The model under review builds one solid part; all positions refer to its coordinate system, in mm. A direction names the side the tool comes from. Coordinates: 2 decimals unless noted, no trailing zeros. Order: outer loops, then holes, each group sorted by start corner. A loop starts at its lowest first (then second) coordinate and runs counter-clockwise, first axis right, second up. Notation, with made-up numbers: (33, 20) -> (63, 20) arc R19 cw to (63, 33) -> close; hole circle Ø2 at (35, 63.5). An arc over 180 degrees is marked (long way). Use one line per item in the form item = value. Start each with the question number.
(1) Take a section at A-A (y = 15.5). State the section outline as (x, z) points, then the cut area to 3 significant figures.
(2) Take a section at D-D (y = 10.25). State the section outline as (x, z) points.
(3) Wall thickness on line 1 along Y through (x, z) = (-21, 2.3); line 2 along X through (y, z) = (0, 1.9); line 3 along X through (y, z) = (-3.5, 1.65): over which ranges is each line inside the solid? List them lowest first.
(4) Take a section at C-C (x = -6). State the section outline as (y, z) points.
(5) Take a section at B-B (z = 1.85). State the section outline as (x, y) points.
(6) For faces 5 (the flat face through (-16.627, 16, 2)), 6 (the flat face through (-5.627, 16, 2)), 7 (the flat face through (-20.127, 9, 1)), list the 3-axis set-ups (+Z, -Z, +X, -X, +Y, -Y) from which the entire face can be reached by the end or side of a thin tool; tool diameter is ignored.
(7) Mouldability with a two-part tool opening along Y and no side actions: class faces 1 (the flat face through (-7, 17.93, 2)), 2 (the flat face through (-23.127, 14, 1)), 3 (the flat face through (-22, -5.61, 1)), 4 (the flat face through (-22, 0.39, 1)) as +Y half, -Y half, draft (parallel to the pull), parting line (faces both ways), or undercut.
(8) Insertion check: pin 1 Ø0.9 at (y, z) = (16, 1) entering from +X; pin 2 Ø4 at (x, y) = (-7.5, 3.5) entering from -Z; pin 3 Ø1.5 at (x, z) = (-13.5, 2) entering from +Y; pin 4 Ø1.5 at (y, z) = (16.5, 2) entering from -X. Each pin has a flat end and moves straight along its axis. Give the tip position at first contact, or say it passes through.
```python
from build123d import *

# Parameters (mm, degrees)
BOSS_EXTRUDE1_DEPTH = 3
SKETCH2_W           = 3
SKETCH2_H           = 3
BOSS_EXTRUDE2_DEPTH = 3


with BuildPart() as part:
    # Sketch1 → Boss-Extrude1 (new body)
    with BuildSketch(Plane.XY):
        Polygon((-0.126642445, 14.929558907), (-0.126642445, -0.070441093), (-20.126642445, -11.610441093), (-23.126642445, -11.610441093), (-23.126642445, -5.610441093), (-20.126642445, -5.610441093), (-20.126642445, 0.389558907), (-23.126642445, 0.389558907), (-23.126642445, 6.389558907), (-20.126642445, 6.389558907), (-20.126642445, 12.389558907), (-23.126642445, 12.389558907), (-23.126642445, 14.929558907), (-14.126642445, 14.929558907), (-11.126642445, 14.929558907), (-3.126642445, 14.929558907), align=None)
    extrude(amount=BOSS_EXTRUDE1_DEPTH)

    # Sketch2 → Boss-Extrude2 (add)
    with BuildSketch(Plane.XY.offset(3)):
        with Locations((-7.126642445, 16.429558907)):
            Rectangle(SKETCH2_W, SKETCH2_H)
        with Locations((-18.126642445, 16.429558907)):
            Rectangle(SKETCH2_W, SKETCH2_H)
    extrude(amount=-BOSS_EXTRUDE2_DEPTH)


solid = part.part
```
Findings:
q1.outline = (-19.63, 0) -> (-16.63, 0) -> (-16.63, 3) -> (-19.63, 3) -> close; (-8.63, 0) -> (-5.63, 0) -> (-5.63, 3) -> (-8.63, 3) -> close
q1.area = 18.0 mm²
q2.outline = (-20.13, 0) -> (-0.13, 0) -> (-0.13, 3) -> (-20.13, 3) -> close
q3.line_1 = -11.61 to -5.61, 0.39 to 6.39, 12.39 to 14.93
q3.line_2 = -20.13 to -0.13
q3.line_3 = -20.13 to -6.07
q4.outline = (-3.46, 0) -> (17.93, 0) -> (17.93, 3) -> (-3.46, 3) -> close
q5.outline = (-23.13, -11.61) -> (-20.13, -11.61) -> (-0.13, -0.07) -> (-0.13, 14.93) -> (-5.63, 14.93) -> (-5.63, 17.93) -> (-8.63, 17.93) -> (-8.63, 14.93) -> (-16.63, 14.93) -> (-16.63, 17.93) -> (-19.63, 17.93) -> (-19.63, 14.93) -> (-23.13, 14.93) -> (-23.13, 12.39) -> (-20.13, 12.39) -> (-20.13, 6.39) -> (-23.13, 6.39) -> (-23.13, 0.39) -> (-20.13, 0.39) -> (-20.13, -5.61) -> (-23.13, -5.61) -> close
q6.face_5 = +Z, -Z, +Y
q6.face_6 = +Z, -Z, +X, +Y
q6.face_7 = +Z, -Z, -X
q7.face_1 = +Y half
q7.face_2 = draft
q7.face_3 = undercut
q7.face_4 = undercut
q8.pin_1 = -5.63
q8.pin_2 = 0
q8.pin_3 = 14.93
q8.pin_4 = -19.63
